The listing builds one solid part. Answer for the finished solid, in the listing's coordinates (mm). Face numbers are marked on the shaded views. Coordinates: 2 decimals unless noted, no trailing zeros. Loops run counter-clockwise (first coordinate to the right, second up) from the corner with the lowest first, then second, coordinate; pieces in that order, holes last. Notation, with made-up numbers: (-16.75, 33) - (-6.75, 33) arc R23 cw to (-6.75, 51) - close; hole circle Ø1 at (78, -12.75). An arc over 180 degrees is marked (long way). Write each question's results on one line, items separated by ' | '. Start each with the question number.
(1) Find section B-B on z = -4. Determine the outline of the cut face in (x, y).
(2) Consider line 1 (Y direction, x = -1.75, z = -9); line 2 (Z direction, x = 4.5, y = 0.5); line 3 (Z direction, x = -4.25, y = 0.5). Determine where each line is inside the solid, lowest interval first. Write a range as from..to.
(3) Determine the mould class of the marked faces 1 and 2 for opening direction X: released by +X, released by -X, zero draft, split by the parting line, or undercut.
(4) Find section A-A on z = -6.75. Determine the outline of the cut face in (x, y).
(5) Find section C-C on z = -10.25. Determine the outline of the cut face in (x, y), then the cut area to 3 significant figures.
(6) Given pin 1 Ø0.8 at (x, z) = (-2.5, -4) entering from +Y; pin 2 Ø6 at (y, z) = (-2.5, -5.5) entering from -X; pin 3 Ø1 at (x, z) = (-0.5, -6) entering from -Y; pin 4 Ø1 at (y, z) = (3, -6.5) entering from +X, each flat-ended and moving along its own axis, determine where each tip first touches the part or whether it passes through.
from build123d import *

# Parameters (mm, degrees)
F3_DEPTH = 10


with BuildPart() as f1:
    # F0 (on Front) → F1 (revolve)
    with BuildSketch(Plane.XZ):
        with BuildLine():
            Line((0, 0), (0, -13.5))
            ThreePointArc((0, -13.5), (6.75, -6.75), (0, 0))
        make_face()
    revolve(axis=Axis((0, 0, -6.75), (0, 0, -1)))

    # F2 (on Top) → F3 (cut)
    with BuildSketch(Plane.XY):
        with BuildLine():
            Line((-3.1, 1.65), (-3.1, 0))
            Line((-3.1, 0), (-3.1, -1.65))
            Line((-3.1, -1.65), (-2.15, -1.65))
            ThreePointArc((-2.15, -1.65), (-1.796447, -1.796447), (-1.65, -2.15))
            Line((-1.65, -2.15), (-1.65, -3.1))
            Line((-1.65, -3.1), (0, -3.1))
            Line((0, -3.1), (1.65, -3.1))
            Line((1.65, -3.1), (1.65, -2.15))
            ThreePointArc((1.65, -2.15), (1.796447, -1.796447), (2.15, -1.65))
            Line((2.15, -1.65), (3.1, -1.65))
            Line((3.1, -1.65), (3.1, 0))
            Line((3.1, 0), (3.1, 1.65))
            Line((3.1, 1.65), (2.15, 1.65))
            ThreePointArc((2.15, 1.65), (1.796447, 1.796447), (1.65, 2.15))
            Line((1.65, 2.15), (1.65, 3.1))
            Line((1.65, 3.1), (0, 3.1))
            Line((0, 3.1), (-1.65, 3.1))
            Line((-1.65, 3.1), (-1.65, 2.15))
            ThreePointArc((-1.65, 2.15), (-1.796447, 1.796447), (-2.15, 1.65))
            Line((-2.15, 1.65), (-3.1, 1.65))
        make_face()
    extrude(amount=-F3_DEPTH, mode=Mode.SUBTRACT)

    # F4 (on Front) → F5 (revolve)
    with BuildSketch(Plane.XZ):
        with BuildLine():
            Line((-6, -13), (-6, -13.5))
            Line((-6, -13.5), (0, -13.5))
            Line((0, -13.5), (0, -12.090374))
            Line((0, -12.090374), (-4.128305, -12.090374))
            ThreePointArc((-4.128305, -12.090374), (-5.037623, -12.599775), (-6, -13))
        make_face()
    revolve(axis=Axis((0, 0, -12.795187), (0, 0, 1)))


solid = f1.part
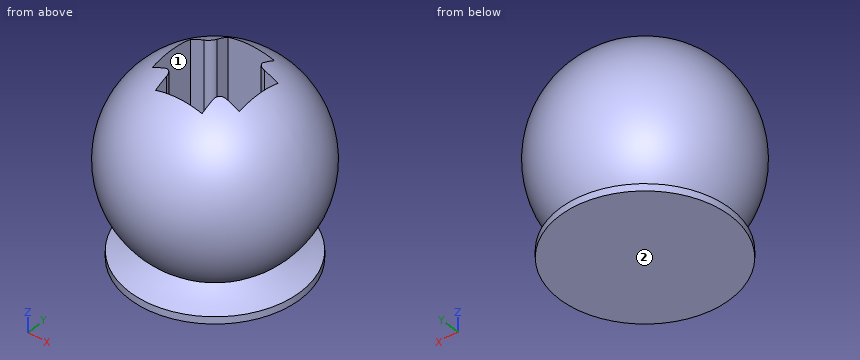
Values:
1) outline: circle Ø12.33 at (0, 0); hole (-3.1, -1.65) - (-2.15, -1.65) arc R0.5 cw to (-1.65, -2.15) - (-1.65, -3.1) - (1.65, -3.1) - (1.65, -2.15) arc R0.5 cw to (2.15, -1.65) - (3.1, -1.65) - (3.1, 1.65) - (2.15, 1.65) arc R0.5 cw to (1.65, 2.15) - (1.65, 3.1) - (-1.65, 3.1) - (-1.65, 2.15) arc R0.5 cw to (-2.15, 1.65) - (-3.1, 1.65) - close
2) line 1: y = -6.12..-1.85, 1.85..6.12 | line 2: z = -13.5..-12.33, -11.76..-1.74 | line 3: z = -13.5..-12.18, -11.97..-1.53
3) face 1: undercut | face 2: zero draft
4) outline: circle Ø13.5 at (0, 0); hole (-3.1, -1.65) - (-2.15, -1.65) arc R0.5 cw to (-1.65, -2.15) - (-1.65, -3.1) - (1.65, -3.1) - (1.65, -2.15) arc R0.5 cw to (2.15, -1.65) - (3.1, -1.65) - (3.1, 1.65) - (2.15, 1.65) arc R0.5 cw to (1.65, 2.15) - (1.65, 3.1) - (-1.65, 3.1) - (-1.65, 2.15) arc R0.5 cw to (-2.15, 1.65) - (-3.1, 1.65) - close
5) outline: circle Ø11.54 at (0, 0) | area: 105 mm²
6) pin 1: stops at y = 5.88 | pin 2: stops at x = -6.75 | pin 3: stops at y = -6.74 | pin 4: stops at x = 6.27
